Autodesk Inventor part; units mm, degrees
ref_plane "YZ Plane" through (0, 0, 0) normal (1, 0, 0) x (0, 1, 0)
ref_plane "XZ Plane" through (0, 0, 0) normal (0, 1, 0) x (-1, 0, 0)
ref_plane "XY Plane" through (0, 0, 0) normal (0, 0, 1) x (1, 0, 0)
sketch "Sketch1" plane through (0, 0, 0) normal (0, 1, 0) x (-1, 0, 0)
  circle A0 centre (0, 0) radius 9.25
  circle A1 centre (0, 0) radius 2.5
  circle A2 centre (0, 0) radius 6.1
  dimension "d0" = 18.5
  dimension "d1" = 5
  dimension "d4" = 12.2
extrude "Extrusion1" add sketch "Sketch1" along normal blind 1 contours A0 | A2
ref_plane "Work Plane1" through (0, 13, 0) normal (0, -1, 0) x (1, 0, 0)
sketch "Sketch2" plane through (0, 13, 0) normal (0, -1, 0) x (1, 0, 0)
  circle A0 centre (0, 0) radius 9.25
  circle A1 centre (0, 0) radius 2.5
extrude "Extrusion2" add sketch "Sketch2" along normal blind 1
extrude "Extrusion3" add sketch "Sketch1" along normal up to surface (12 mm away) contours A2
properties part number "Idler Pulley 10mm 5mm Bore" material "Aluminum 6061"
Source: CAD feature listing. Evaluate the final solid. Frame: model axes, mm. A direction names the side the tool comes from. Round coordinates to 2 decimals unless told otherwise and drop trailing zeros. Loops run counter-clockwise (first coordinate to the right, second up) from the corner with the lowest first, then second, coordinate; pieces in that order, holes last.
Q1. Access query for faces 4 (the face through (-2, 0, -2)), 5 (the face through (-6, 1, -2)). Directions: +Z, -Z, +X, -X, +Y, -Y. A direction counts if a zero-diameter tool reaches every point of the face in a straight line with its end or side. Return the directions, or none.
Q2. Section D-D, the plane x = -5.5. Return loops of the section in (y, z).
Q3. Mould query, pull axis Y, two halves, no side actions, for faces 1 (the face through (6.094, 6.423, -0.268)), 2 (the face through (-2.01, 12.51, 9.03)), 3 (the face through (2, 13, -2)). Classes: pulls with the +Y half, pulls with the -Y half, needs draft (parallel to the pull), parting line crosses it, or undercut.
Q4. First-contact query: P1, Ø6, axis at y = 10, z = -3, coming from the +X side; P2, Ø6, axis at x = 6.5, y = 7.5, coming from the +Z side; P3, Ø5, axis at x = -7, y = 4, coming from the +Z side; P4, Ø4, axis at x = -4, z = -6.5, coming from the -Y side. Flat tips, straight axial feed; report the tip coordinate or a pass-through.
Q5. Section B-B, the plane y = 3.5. Return loops of the section in (x, z).
Q6. Ray query, line 1 (X direction, y = 5, z = 0); line 2 (Y direction, x = -2.5, z = 6.5). Return the intervals inside material, ascending.
Q7. Section C-C, the plane x = 4.5. Return loops of the section in (y, z), plus the area to 3 significant figures.
Solutions:
1. face 4: +Z, -Z, +X, -X, -Y
1. face 5: none
2. outline: (0, -7.44) - (1, -7.44) - (1, -2.64) - (12, -2.64) - (12, -7.44) - (13, -7.44) - (13, 7.44) - (12, 7.44) - (12, 2.64) - (1, 2.64) - (1, 7.44) - (0, 7.44) - close
3. face 1: undercut
3. face 2: needs draft
3. face 3: pulls with the +Y half
4. P1: stops at x = 9.22
4. P2: stops at z = 5
4. P3: stops at z = 4.12
4. P4: stops at y = 0
5. outline: circle Ø12.2 at (0, 0); hole circle Ø5 at (0, 0)
6. line 1: x = -6.1 to -2.5, 2.5 to 6.1
6. line 2: y = 0 to 1, 12 to 13
7. outline: (0, -8.08) - (1, -8.08) - (1, -4.12) - (12, -4.12) - (12, -8.08) - (13, -8.08) - (13, 8.08) - (12, 8.08) - (12, 4.12) - (1, 4.12) - (1, 8.08) - (0, 8.08) - close
7. area: 123 mm2
